Read the model definition and answer for the solid it produces. Units are mm, in the model's axes. A direction names the side the tool comes from. Give positions to 0.01 mm unless a question says otherwise; leave off trailing zeros. Write each loop counter-clockwise with the first axis right and the second up, starting at its lowest first coordinate (ties: lowest second). Pieces come first, ordered by that corner, then holes. Notation, with made-up numbers: (30.5, -9.75) - (76.5, -9.75) arc R18 ccw to (76.5, 22.25) - close; hole circle Ø10 at (40, 38.5). An arc over 180 degrees is marked (long way). Answer as a JSON object with one key per item and string values. Group by question number.
```python
from build123d import *

# Parameters (mm, degrees)
BOSS_EXTRUDE1_DEPTH = 12.7
SKETCH2_R           = 3.571875
BOSS_EXTRUDE2_DEPTH = 6.35


with BuildPart() as part:
    # Sketch1 → Boss-Extrude1 (new body)
    with BuildSketch(Plane(origin=(0, 0, 0), x_dir=(1, 0, 0), z_dir=(0, 1, 0))):
        Polygon((0, 0), (25.4, 0), (33.3375, -5.265141855), (33.3375, -17.965141855), (29.395430976, -20.6375), (8.757930976, -20.6375), (4.267802915, -19.05), (0, -14.2875), align=None)
    extrude(amount=BOSS_EXTRUDE1_DEPTH)

    # Sketch2 → Boss-Extrude2 (add)
    with BuildSketch(Plane(origin=(33.3375, 0, 0), x_dir=(0, 0, -1), z_dir=(1, 0, 0))):
        with Locations((-9.614891855, 6.35)):
            Circle(SKETCH2_R)
    extrude(amount=BOSS_EXTRUDE2_DEPTH)


solid = part.part
```
1) Find the intervals of material crossed by line 1 (X direction, y = 11, z = 3.5); line 2 (X direction, y = 1.75, z = 1); line 3 (Z direction, x = 33, y = 6.5), in increasing order. Write a range as [from, to].
2) Find section A-A, the plane y = 6.35. Write down the section's boundary in (x, z).
3) Which of the six approach directions +Z, -Z, +X, -X, +Y, -Y give full straight-line access (tool end or side, diameter ignored) to faces 1 (the cylindrical face through (36.47, 9.89, 10.08)), 2 (the flat face through (17, 12.7, 10))?
4) Find section D-D, the plane x = 26. Write down the section's boundary in (y, z), and give its area (3 significant figures).
5) Find section B-B, the plane z = 11. Write down the section's boundary in (x, y).
6) Find section C-C, the plane y = 11.25. Write down the section's boundary in (x, z).
Values follow:
{
 "1": {"line 1": "x = [0, 30.68]", "line 2": "x = [0, 26.91]", "line 3": "z = [5.04, 18.19]"},
 "2": {"outline": "(0, 0) - (25.4, 0) - (33.34, 5.27) - (33.34, 6.04) - (39.69, 6.04) - (39.69, 13.19) - (33.34, 13.19) - (33.34, 17.97) - (29.4, 20.64) - (8.76, 20.64) - (4.27, 19.05) - (0, 14.29) - close"},
 "3": {"face 1": "+X", "face 2": "+Z, -Z, +X, -X, +Y"},
 "4": {"outline": "(0, 0.4) - (12.7, 0.4) - (12.7, 20.64) - (0, 20.64) - close", "area": "257 mm2"},
 "5": {"outline": "(0, 0) - (33.34, 0) - (33.34, 3.06) - (39.69, 3.06) - (39.69, 9.64) - (33.34, 9.64) - (33.34, 12.7) - (0, 12.7) - close"},
 "6": {"outline": "(0, 0) - (25.4, 0) - (33.34, 5.27) - (33.34, 17.97) - (29.4, 20.64) - (8.76, 20.64) - (4.27, 19.05) - (0, 14.29) - close"}
}
